Geometry: final body of the model. Coordinates: model frame, mm. Give positions to 0.01 mm unless a question says otherwise; leave off trailing zeros. Write each loop counter-clockwise with the first axis right and the second up, starting at its lowest first coordinate (ties: lowest second). Pieces come first, ordered by that corner, then holes. Notation, with made-up numbers: M 79.25,52.25 L 109.25,52.25 A17 cw 109.25,85.25 Z; hole C -27.75,-11 d9. An arc over 180 degrees is marked long. Use a Markdown table: item, result. Add a question column.
1) Section B-B on z = 68. Return the cut outline in (x, y).
2) Pin query (flat end, axial travel): pin 1 (3.5 mm diameter, centred on x = -29, z = -17, fed in from -Y). Return the tip coordinate at first contact, or that it passes through.
3) Section D-D on x = 49. Return the cut outline in (y, z).
4) Section A-A on x = 119. Return the cut outline in (y, z), then the cut area to 3 significant figures.
5) Section C-C on y = 0.7. State how many separate pieces and enclosed holes the cut face has, then the cut area to 3 significant figures.
6) Line query: line 1 (X direction, y = -0.1, z = -42); line 2 (Z direction, x = 49, y = 0.35); line 3 (X direction, y = -0.2, z = -22). Output: solid intervals per line, ascending.
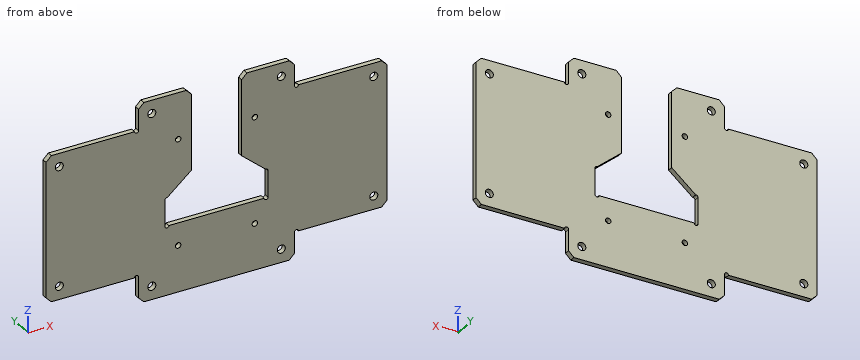
```python
from build123d import *

# Parameters (mm, degrees)
SKETCH_1_R          = 3.05
EXTRUDE_1_DEPTH     = 2
CUT_EXTRUDE_1_DEPTH = 163.052460642
SKETCH_3_R          = 1.5
CUT_EXTRUDE_2_DEPTH = 163.052460642
SKETCH_4_R          = 2.05
CUT_EXTRUDE_3_DEPTH = 163.052460642
CHAMFER_1_SIZE      = 4


with BuildPart() as part:
    # 草图1 → 凸台-拉伸1 (new, symmetric)
    with BuildSketch(Plane(origin=(0, 0, 0), x_dir=(1, 0, 0), z_dir=(0, 1, 0))):
        Polygon((59, 52), (-59, 52), (-59, 32), (-129, 32), (-129, -78), (-59, -78), (-59, -98), (-19, -98), (-19, 0), (19, 0), (19, -98), (59, -98), (59, -78), (129, -78), (129, 32), (59, 32), align=None)
        with Locations(Location((-49, 42, 0), (0, 0, 270))):
            Circle(SKETCH_1_R, mode=Mode.SUBTRACT)
        with Locations(Location((-119, 22, 0), (0, 0, 270))):
            Circle(SKETCH_1_R, mode=Mode.SUBTRACT)
        with Locations(Location((-119, -68, 0), (0, 0, 270))):
            Circle(SKETCH_1_R, mode=Mode.SUBTRACT)
        with Locations(Location((-49, -88, 0), (0, 0, 270))):
            Circle(SKETCH_1_R, mode=Mode.SUBTRACT)
        with Locations(Location((49, -88, 0), (0, 0, 90))):
            Circle(SKETCH_1_R, mode=Mode.SUBTRACT)
        with Locations(Location((119, -68, 0), (0, 0, 90))):
            Circle(SKETCH_1_R, mode=Mode.SUBTRACT)
        with Locations(Location((119, 22, 0), (0, 0, 90))):
            Circle(SKETCH_1_R, mode=Mode.SUBTRACT)
        with Locations(Location((49, 42, 0), (0, 0, 90))):
            Circle(SKETCH_1_R, mode=Mode.SUBTRACT)
    extrude(amount=EXTRUDE_1_DEPTH, both=True)

    # 草图2 → 切除-拉伸1 (cut, through all)
    with BuildSketch(Plane(origin=(0, 2, 0), x_dir=(1, 0, 0), z_dir=(0, 1, 0))):
        Polygon((-19, 0), (-39, 0), (-39, -20), (-19, -36.781992624), align=None)
        Polygon((39, -20), (19, -36.781992624), (19, 0), (39, 0), align=None)
    extrude(amount=-CUT_EXTRUDE_1_DEPTH, mode=Mode.SUBTRACT)

    # 草图3 → 切除-拉伸2 (cut, through all)
    with BuildSketch(Plane(origin=(0, 2, 0), x_dir=(1, 0, 0), z_dir=(0, 1, 0))):
        with Locations((-37.5, 0)):
            Circle(SKETCH_3_R)
        with Locations((-37.5, -20)):
            Circle(SKETCH_3_R)
        with Locations((37.5, -20)):
            Circle(SKETCH_3_R)
        with Locations((37.5, 0)):
            Circle(SKETCH_3_R)
        with Locations((-60.5, 32)):
            Circle(SKETCH_3_R)
        with Locations((-60.5, -78)):
            Circle(SKETCH_3_R)
        with Locations((60.5, -78)):
            Circle(SKETCH_3_R)
        with Locations((60.5, 32)):
            Circle(SKETCH_3_R)
    extrude(amount=-CUT_EXTRUDE_2_DEPTH, mode=Mode.SUBTRACT)

    # 草图4 → 切除-拉伸3 (cut, through all)
    with BuildSketch(Plane(origin=(0, 2, 0), x_dir=(1, 0, 0), z_dir=(0, 1, 0))):
        with Locations(Location((-29, -63, 0), (0, 0, 270))):
            Circle(SKETCH_4_R)
        with Locations(Location((29, -63, 0), (0, 0, 270))):
            Circle(SKETCH_4_R)
        with Locations(Location((29, 17, 0), (0, 0, 270))):
            Circle(SKETCH_4_R)
        with Locations(Location((-29, 17, 0), (0, 0, 270))):
            Circle(SKETCH_4_R)
    extrude(amount=-CUT_EXTRUDE_3_DEPTH, mode=Mode.SUBTRACT)

    # 倒角1
    chamfer_1_edges = [part.edges().sort_by_distance(p)[0] for p in [
        (-129, 0, 78),
        (-129, 0, -32),
        (-59, 0, -52),
        (59, 0, -52),
        (129, 0, -32),
        (129, 0, 78),
        (59, 0, 98),
        (19, 0, 98),
        (-19, 0, 98),
        (-59, 0, 98),
    ]]
    chamfer(chamfer_1_edges, length=CHAMFER_1_SIZE)


solid = part.part
```
Found:
| question | item | result |
|---|---|---|
| 1 | outline | M -129,-2 L -122.05,-2 L -122.05,2 L -129,2 Z; M -115.95,-2 L -19,-2 L -19,2 L -115.95,2 Z; M 19,-2 L 115.95,-2 L 115.95,2 L 19,2 Z; M 122.05,-2 L 129,-2 L 129,2 L 122.05,2 Z |
| 2 | pin 1 | through |
| 3 | outline | M -2,-52 L 2,-52 L 2,-45.05 L -2,-45.05 Z; M -2,-38.95 L 2,-38.95 L 2,84.95 L -2,84.95 Z; M -2,91.05 L 2,91.05 L 2,98 L -2,98 Z |
| 4 | outline | M -2,-32 L 2,-32 L 2,-25.05 L -2,-25.05 Z; M -2,-18.95 L 2,-18.95 L 2,64.95 L -2,64.95 Z; M -2,71.05 L 2,71.05 L 2,78 L -2,78 Z |
| 4 | area | 391 mm² |
| 5 | separate pieces | 1 |
| 5 | enclosed holes | 12 |
| 5 | area | 27,900 mm² |
| 6 | line 1 | -59 to -52.05, -45.95 to 45.95, 52.05 to 59 |
| 6 | line 2 | -52 to -45.05, -38.95 to 84.95, 91.05 to 98 |
| 6 | line 3 | -129 to -122.05, -115.95 to 115.95, 122.05 to 129 |
